Design review of the part built by this model. Coordinates are the model's own, in mm. A direction names the side the tool comes from. Coordinates: 2 decimals unless noted, no trailing zeros. Write each loop counter-clockwise with the first axis right and the second up, starting at its lowest first coordinate (ties: lowest second). Pieces come first, ordered by that corner, then holes.
```python
from build123d import *

# Parameters (mm, degrees)
SKETCH1_W                                   = 142.748
SKETCH1_H                                   = 50.8
BOSS_EXTRUDE1_DEPTH                         = 63.5
SHELL1_T                                    = -3.81
SKETCH2_W                                   = 155.448
SKETCH2_H                                   = 3.81
BOSS_EXTRUDE2_DEPTH                         = 6.35
SKETCH3_W                                   = 155.448
SKETCH3_H                                   = 3.81
BOSS_EXTRUDE3_DEPTH                         = 6.35
SKETCH4_W                                   = 50.8
SKETCH4_H                                   = 3.81
BOSS_EXTRUDE4_DEPTH                         = 6.35
SKETCH5_W                                   = 50.8
SKETCH5_H                                   = 3.81
BOSS_EXTRUDE5_DEPTH                         = 6.35
CBORE_FOR_00_BINDING_HEAD_MACHINE_S_2_COUNT = 2
CBORE_FOR_00_BINDING_HEAD_MACHINE_S_2_PITCH = 147.800013628
CBORE_FOR_00_BINDING_HEAD_MACHINE_S_3_COUNT = 2
CBORE_FOR_00_BINDING_HEAD_MACHINE_S_3_PITCH = 158.036995618
CBORE_FOR_00_BINDING_HEAD_MACHINE_S_4_COUNT = 2
CBORE_FOR_00_BINDING_HEAD_MACHINE_S_4_PITCH = 55.88
SKETCH13_W                                  = 135.128
SKETCH13_H                                  = 6.604
BOSS_EXTRUDE6_DEPTH                         = 20.32
SKETCH14_R                                  = 4.072823047
CUT_EXTRUDE1_DEPTH                          = 13.97


with BuildPart() as part:
    # Sketch1 → Boss-Extrude1 (new body)
    with BuildSketch(Plane(origin=(0, 0, 0), x_dir=(1, 0, 0), z_dir=(0, 1, 0))):
        with Locations((71.374, 25.4)):
            Rectangle(SKETCH1_W, SKETCH1_H)
    extrude(amount=BOSS_EXTRUDE1_DEPTH)

    # Shell1
    shell1_openings = [part.faces().sort_by_distance(p)[0] for p in [
        (71.374, 63.5, -25.4),
    ]]
    offset(amount=SHELL1_T, openings=shell1_openings, kind=Kind.INTERSECTION)

    # Sketch2 → Boss-Extrude2 (add)
    with BuildSketch(Plane.XY):
        with Locations((71.374, 61.595)):
            Rectangle(SKETCH2_W, SKETCH2_H)
    extrude(amount=BOSS_EXTRUDE2_DEPTH)

    # Sketch3 → Boss-Extrude3 (add)
    with BuildSketch(Plane(origin=(0, 0, -50.8), x_dir=(-1, 0, 0), z_dir=(0, 0, -1))):
        with Locations((-71.374, 61.595)):
            Rectangle(SKETCH3_W, SKETCH3_H)
    extrude(amount=BOSS_EXTRUDE3_DEPTH)

    # Sketch4 → Boss-Extrude4 (add)
    with BuildSketch(Plane.ZY):
        with Locations((-25.4, 61.595)):
            Rectangle(SKETCH4_W, SKETCH4_H)
    extrude(amount=BOSS_EXTRUDE4_DEPTH)

    # Sketch5 → Boss-Extrude5 (add)
    with BuildSketch(Plane(origin=(142.748, 0, 0), x_dir=(0, 0, -1), z_dir=(1, 0, 0))):
        with Locations((25.4, 61.595)):
            Rectangle(SKETCH5_W, SKETCH5_H)
    extrude(amount=BOSS_EXTRUDE5_DEPTH)

    # Sketch11 → CBORE for #00 Binding Head Machine Screw3 (revolve, cut)
    with BuildSketch(Plane(origin=(-2.54, 59.69, 2.54), x_dir=(0, 0, -1), z_dir=(1, 0, 0))):
        Polygon((0, 0), (0, 3.81), (0.6604, 3.81), (0.6604, 0.7112), (1.5875, 0.7112), (1.5875, 0.532828266), (2.2225, 0), align=None)
    cbore_for_00_binding_head_machine_screw = revolve(axis=Axis((-2.54, 53.34, 2.54), (0, 1, 0)), mode=Mode.SUBTRACT)

    # CBORE for _00 Binding Head Machine S 2: CBORE for #00 Binding Head Machine Screw3 ×2
    with Locations(*[(i * CBORE_FOR_00_BINDING_HEAD_MACHINE_S_2_PITCH, 0, 0) for i in range(1, CBORE_FOR_00_BINDING_HEAD_MACHINE_S_2_COUNT)]):
        add(cbore_for_00_binding_head_machine_screw, mode=Mode.SUBTRACT)

    # CBORE for _00 Binding Head Machine S 3: CBORE for #00 Binding Head Machine Screw3 ×2
    with Locations(*[Vector(0.9354012294514634, 0, -0.35358809360708243) * (i * CBORE_FOR_00_BINDING_HEAD_MACHINE_S_3_PITCH) for i in range(1, CBORE_FOR_00_BINDING_HEAD_MACHINE_S_3_COUNT)]):
        add(cbore_for_00_binding_head_machine_screw, mode=Mode.SUBTRACT)

    # CBORE for _00 Binding Head Machine S 4: CBORE for #00 Binding Head Machine Screw3 ×2
    with Locations(*[(0, 0, -i * CBORE_FOR_00_BINDING_HEAD_MACHINE_S_4_PITCH) for i in range(1, CBORE_FOR_00_BINDING_HEAD_MACHINE_S_4_COUNT)]):
        add(cbore_for_00_binding_head_machine_screw, mode=Mode.SUBTRACT)

    # Sketch13 → Boss-Extrude6 (add)
    with BuildSketch(Plane(origin=(0, 3.81, 0), x_dir=(1, 0, 0), z_dir=(0, 1, 0))):
        with Locations((71.374, 43.688)):
            Rectangle(SKETCH13_W, SKETCH13_H)
        with Locations((71.374, 7.112)):
            Rectangle(SKETCH13_W, SKETCH13_H)
    extrude(amount=BOSS_EXTRUDE6_DEPTH)

    # Sketch14 → Cut-Extrude1 (cut)
    with BuildSketch(Plane.XY):
        with Locations((12.280475356, 11.107728565)):
            Circle(SKETCH14_R)
    extrude(amount=-CUT_EXTRUDE1_DEPTH, mode=Mode.SUBTRACT)


solid = part.part
```
(1) Insertion check: pin 1 Ø12 at (x, y) = (88.5, 49) entering from +Z; pin 2 Ø6 at (x, z) = (79, -43.5) entering from +Y; pin 3 Ø12 at (x, y) = (71.5, 43) entering from -Z; pin 4 Ø4 at (x, z) = (-2.54, -53.34) entering from +Y. Each pin has a flat end and moves straight along its axis. Give the tip position at first contact, or say it passes through.
(2) Consider section C-C (z = -8.5). Give the boundary of the cut face in (x, y).
(3) Consider section A-A (x = 130). Give the boundary of the cut face in (y, z), plus the area to 3 significant figures.
(4) For faces 4 (the flat face through (149.098, 62, -25)), 5 (the flat face through (138.938, 33, -25)), list the 3-axis set-ups (+Z, -Z, +X, -X, +Y, -Y) from which the entire face can be reached by the end or side of a thin tool; tool diameter is ignored.
(5) Consider section B-B (y = 43.5). Give the boundary of the cut face in (x, z), plus the area to 3 significant figures.
(6) Mouldability with a two-part tool opening along Z and no side actions: class faces 1 (the flat face through (70, 14, -40.386)), 2 (the cylindrical face through (11.4, 7.13, -5.13)), 3 (the flat face through (70, 29, 0)) as +Z half, -Z half, draft (parallel to the pull), parting line (faces both ways), or undercut.
(7) Wall thickness on line 1 (X direction, y = 60.3, z = -53.34); line 2 (Z direction, x = 98, y = 43); line 3 (Z direction, x = 84.5, y = 61): over which ranges is each line inside the solid? List them lowest first.
(8) Consider section D-D (x = 12). Give the boundary of the cut face in (y, z).
Results:
1. pin 1: stops at z = 0
1. pin 2: stops at y = 24.13
1. pin 3: stops at z = -50.8
1. pin 4: stops at y = 63.5
2. outline: (-6.35, 59.69) - (0, 59.69) - (0, 0) - (142.75, 0) - (142.75, 59.69) - (149.1, 59.69) - (149.1, 63.5) - (138.94, 63.5) - (138.94, 24.13) - (3.81, 24.13) - (3.81, 63.5) - (-6.35, 63.5) - close; hole circle Ø8.15 at (12.28, 11.11)
3. outline: (0, -50.8) - (59.69, -50.8) - (59.69, -57.15) - (63.5, -57.15) - (63.5, -46.99) - (24.13, -46.99) - (24.13, -40.39) - (3.81, -40.39) - (3.81, -10.41) - (24.13, -10.41) - (24.13, -3.81) - (63.5, -3.81) - (63.5, 6.35) - (59.69, 6.35) - (59.69, 0) - (0, 0) - close
3. area: 965 mm2
4. face 4: +Z, -Z, +X, +Y, -Y
4. face 5: +Y
5. outline: (0, -50.8) - (142.75, -50.8) - (142.75, 0) - (0, 0) - close; hole (3.81, -46.99) - (138.94, -46.99) - (138.94, -3.81) - (3.81, -3.81) - close
5. area: 1,420 mm2
6. face 1: undercut
6. face 2: draft
6. face 3: +Z half
7. line 1: x = -6.35 to -4.13, -0.95 to 143.7, 146.88 to 149.1
7. line 2: z = -50.8 to -46.99, -3.81 to 0
7. line 3: z = -57.15 to -46.99, -3.81 to 6.35
8. outline: (0, -50.8) - (59.69, -50.8) - (59.69, -57.15) - (63.5, -57.15) - (63.5, -46.99) - (24.13, -46.99) - (24.13, -40.39) - (3.81, -40.39) - (3.81, -10.41) - (7.04, -10.41) - (7.04, 0) - (0, 0) - close; (15.17, -10.41) - (24.13, -10.41) - (24.13, -3.81) - (63.5, -3.81) - (63.5, 6.35) - (59.69, 6.35) - (59.69, 0) - (15.17, 0) - close
